Work out the finished part from the listing and answer in its coordinate system (mm). A direction names the side the tool comes from. Round coordinates to 2 decimals unless told otherwise and drop trailing zeros. Write each loop counter-clockwise with the first axis right and the second up, starting at its lowest first coordinate (ties: lowest second). Pieces come first, ordered by that corner, then holes. Notation, with made-up numbers: (39.5, 7) -> (47.5, 7) arc R28 cw to (47.5, 41) -> close; hole circle Ø5 at (55.25, 46.5). An arc over 180 degrees is marked (long way). Answer as a JSON object with one key per item and string values. Group by question number.
from build123d import *

# Parameters (mm, degrees)
SKETCH_1_W               = 5.5
SKETCH_1_H               = 9.9
EXTRUDE_1_DEPTH          = 6.44
SKETCH_2_W               = 1.5
SKETCH_2_H               = 0.15
PATTERN_LINEAR_1_COUNT   = 2
PATTERN_LINEAR_1_PITCH   = 2.54
SKETCH_3_W               = 1.5
SKETCH_3_H               = 0.15
PATTERN_LINEAR_2_COUNT   = 2
PATTERN_LINEAR_2_PITCH   = 2.54
CUT_EXTRUDE_1_DEPTH      = 0.15
CUT_EXTRUDE_1_DEPTH_BACK = 0.15
CUT_EXTRUDE_4_DEPTH      = 0.15
CUT_EXTRUDE_4_DEPTH_BACK = 0.15
CUT_EXTRUDE_5_DEPTH      = 0.15
CUT_EXTRUDE_5_DEPTH_BACK = 0.15
CUT_EXTRUDE_6_DEPTH      = 0.15
CUT_EXTRUDE_6_DEPTH_BACK = 0.15
SKETCH_6_W               = 1.4
SKETCH_6_H               = 3.5
CUT_EXTRUDE_1_2_DEPTH    = 1
PATTERN_LINEAR_3_COUNT   = 2
PATTERN_LINEAR_3_PITCH   = 2.54
EXTRUDE_2_DEPTH          = 2
SKETCH_8_W               = 5.49587381
SKETCH_8_H               = 0.4
EXTRUDE_3_DEPTH          = 0.4
FILLET_1_R               = 0.08


with BuildPart() as part:
    # Эскиз1 → Вытянуть1 (new body)
    with BuildSketch(Plane(origin=(0, 0, 0), x_dir=(0, 0, -1), z_dir=(1, 0, 0))):
        Rectangle(SKETCH_1_W, SKETCH_1_H)
    extrude(amount=EXTRUDE_1_DEPTH)

    # По траектории1: sweep along a curve in space
    with BuildLine() as sweep_1_path:
        Line((4.49, 3.95, -2.75), (4.49, 3.95, -3.790830974))
        ThreePointArc((4.49, 3.95, -3.790830974), (4.49, 3.906490428, -3.915373119), (4.49, 3.794892541, -3.98572751))
        Line((4.49, 3.794892541, -3.98572751), (4.49, -3.95, -5.769688961))
        Line((4.49, -3.95, -5.769688961), (4.49, -7.85, -5.769688961))
    # Эскиз2 → По траектории1 (sweep)
    with BuildSketch(Plane(origin=(0, 0, -2.75), x_dir=(-1, 0, 0), z_dir=(0, 0, -1))):
        with Locations((-4.49, 3.95)):
            Rectangle(SKETCH_2_W, SKETCH_2_H)
    sweep_1 = sweep(path=sweep_1_path.line, transition=Transition.RIGHT)

    # Линейный массив1: По траектории1 ×2
    with Locations(*[(-i * PATTERN_LINEAR_1_PITCH, 0, 0) for i in range(1, PATTERN_LINEAR_1_COUNT)]):
        add(sweep_1)

    # По траектории2: sweep along a curve in space
    with BuildLine() as sweep_2_path:
        Line((4.49, -3.95, -2.75), (4.49, -3.95, -4.02144183))
        ThreePointArc((4.49, -3.95, -4.02144183), (4.49, -4.008578644, -4.162863187), (4.49, -4.15, -4.22144183))
        Line((4.49, -4.15, -4.22144183), (4.49, -7.85, -4.22144183))
    # Эскиз3 → По траектории2 (sweep)
    with BuildSketch(Plane(origin=(0, 0, -2.75), x_dir=(-1, 0, 0), z_dir=(0, 0, -1))):
        with Locations((-4.49, -3.95)):
            Rectangle(SKETCH_3_W, SKETCH_3_H)
    sweep_2 = sweep(path=sweep_2_path.line)

    # Линейный массив2: По траектории2 ×2
    with Locations(*[(-i * PATTERN_LINEAR_2_PITCH, 0, 0) for i in range(1, PATTERN_LINEAR_2_COUNT)]):
        add(sweep_2)

    # Эскиз4 → Cut-Extrude 1 (cut, two sides: drawn at the far end of the back side and taken through both)
    with BuildSketch(Plane(origin=(0, 0, -5.844688961), x_dir=(-1, 0, 0), z_dir=(0, 0, -1)).offset(-CUT_EXTRUDE_1_DEPTH_BACK)):
        Polygon((-1.21347651, -4.143413371), (-1.665, -5.067248723), (-1.665, -6.848447142), (-1.871476359, -7.835), (-2.028523641, -7.835), (-2.235, -6.848447142), (-2.235, -5.067248723), (-2.68652349, -4.143413371), (-2.71347651, -4.156586629), (-2.265, -5.074187736), (-2.265, -6.851552858), (-2.052894917, -7.865), (-1.847105083, -7.865), (-1.635, -6.851552858), (-1.635, -5.074187736), (-1.18652349, -4.156586629), align=None)
    extrude(amount=CUT_EXTRUDE_1_DEPTH + CUT_EXTRUDE_1_DEPTH_BACK, mode=Mode.SUBTRACT)


with BuildPart() as cut_extrude_1_kept_piece:
    # of the separate pieces the step leaves, the one the design keeps (cut_extrude_1_pieces_kept)
    add(part.part.solids().sort_by_distance((0, 4.95, 2.75))[0])

    # Эскиз4<4> → Вырез-Вытянуть-Тонкостенный4 (cut, two sides: drawn at the far end of the back side and taken through both)
    with BuildSketch(Plane(origin=(0, 0, -5.844688961), x_dir=(-1, 0, 0), z_dir=(0, 0, -1)).offset(-CUT_EXTRUDE_4_DEPTH_BACK)):
        Polygon((-1.21347651, -4.143413371), (-1.665, -5.067248723), (-1.665, -6.848447142), (-1.871476359, -7.835), (-2.028523641, -7.835), (-2.235, -6.848447142), (-2.235, -5.067248723), (-2.68652349, -4.143413371), (-2.71347651, -4.156586629), (-2.265, -5.074187736), (-2.265, -6.851552858), (-2.052894917, -7.865), (-1.847105083, -7.865), (-1.635, -6.851552858), (-1.635, -5.074187736), (-1.18652349, -4.156586629), align=None)
        Polygon((-5.25347651, -4.156586629), (-4.805, -5.074187736), (-4.805, -6.851558008), (-4.592177182, -7.865), (-4.387822818, -7.865), (-4.175, -6.851558008), (-4.175, -5.074187736), (-3.72652349, -4.156586629), (-3.75347651, -4.143413371), (-4.205, -5.067248723), (-4.205, -6.848441992), (-4.412177182, -7.835), (-4.567822818, -7.835), (-4.775, -6.848441992), (-4.775, -5.067248723), (-5.22652349, -4.143413371), align=None)
    extrude(amount=CUT_EXTRUDE_4_DEPTH + CUT_EXTRUDE_4_DEPTH_BACK, mode=Mode.SUBTRACT)


with BuildPart() as cut_extrude_4_kept_piece:
    # of the separate pieces the step leaves, the one the design keeps (cut_extrude_4_pieces_kept)
    add(cut_extrude_1_kept_piece.part.solids().sort_by_distance((0, 4.95, 2.75))[0])

    # Эскиз5 → Вырез-Вытянуть-Тонкостенный5 (cut, two sides: drawn at the far end of the back side and taken through both)
    with BuildSketch(Plane.XY.offset(-4.14644183).offset(-CUT_EXTRUDE_5_DEPTH_BACK)):
        Polygon((1.18652349, -4.156586629), (1.635, -5.074187736), (1.635, -6.851552858), (1.847105083, -7.865), (2.052894917, -7.865), (2.265, -6.851552858), (2.265, -5.074187736), (2.71347651, -4.156586629), (2.68652349, -4.143413371), (2.235, -5.067248723), (2.235, -6.848447142), (2.028523641, -7.835), (1.871476359, -7.835), (1.665, -6.848447142), (1.665, -5.067248723), (1.21347651, -4.143413371), align=None)
    extrude(amount=CUT_EXTRUDE_5_DEPTH + CUT_EXTRUDE_5_DEPTH_BACK, mode=Mode.SUBTRACT)


with BuildPart() as cut_extrude_5_kept_piece:
    # of the separate pieces the step leaves, the one the design keeps (cut_extrude_5_pieces_kept)
    add(cut_extrude_4_kept_piece.part.solids().sort_by_distance((0, 4.95, 2.75))[0])

    # Эскиз5<4> → Вырез-Вытянуть-Тонкостенный6 (cut, two sides: drawn at the far end of the back side and taken through both)
    with BuildSketch(Plane.XY.offset(-4.14644183).offset(-CUT_EXTRUDE_6_DEPTH_BACK)):
        Polygon((1.18652349, -4.156586629), (1.635, -5.074187736), (1.635, -6.851552858), (1.847105083, -7.865), (2.052894917, -7.865), (2.265, -6.851552858), (2.265, -5.074187736), (2.71347651, -4.156586629), (2.68652349, -4.143413371), (2.235, -5.067248723), (2.235, -6.848447142), (2.028523641, -7.835), (1.871476359, -7.835), (1.665, -6.848447142), (1.665, -5.067248723), (1.21347651, -4.143413371), align=None)
        Polygon((5.22652349, -4.143413371), (4.775, -5.067248723), (4.775, -6.848441992), (4.567822818, -7.835), (4.412177182, -7.835), (4.205, -6.848441992), (4.205, -5.067248723), (3.75347651, -4.143413371), (3.72652349, -4.156586629), (4.175, -5.074187736), (4.175, -6.851558008), (4.387822818, -7.865), (4.592177182, -7.865), (4.805, -6.851558008), (4.805, -5.074187736), (5.25347651, -4.156586629), align=None)
    extrude(amount=CUT_EXTRUDE_6_DEPTH + CUT_EXTRUDE_6_DEPTH_BACK, mode=Mode.SUBTRACT)


with BuildPart() as cut_extrude_6_kept_piece:
    # of the separate pieces the step leaves, the one the design keeps (cut_extrude_6_pieces_kept)
    add(cut_extrude_5_kept_piece.part.solids().sort_by_distance((0, 4.95, 2.75))[0])

    # Эскиз6 → Cut-Extrude 1 2 (cut)
    with BuildSketch(Plane.XY.offset(2.75)):
        with Locations((2.004611319, 0)):
            Rectangle(SKETCH_6_W, SKETCH_6_H)
    cut_extrude_1_2 = extrude(amount=-CUT_EXTRUDE_1_2_DEPTH, mode=Mode.SUBTRACT)

    # Линейный массив3: Cut-Extrude 1 2 ×2
    with Locations(*[(i * PATTERN_LINEAR_3_PITCH, 0, 0) for i in range(1, PATTERN_LINEAR_3_COUNT)]):
        add(cut_extrude_1_2, mode=Mode.SUBTRACT)

    # Эскиз7 → Вытянуть2 (add)
    with BuildSketch(Plane.XY.offset(1.75)):
        with BuildLine():
            Line((1.304611319, -0.15), (1.304611319, -1.75))
            ThreePointArc((1.304611319, -1.75), (2.004611319, -1.460050506), (2.704611319, -1.75))
            Line((2.704611319, -1.75), (2.704611319, -0.15))
            ThreePointArc((2.704611319, -0.15), (2.004611319, -0.439949494), (1.304611319, -0.15))
        make_face()
        with BuildLine():
            Line((3.844611319, -0.15), (3.844611319, -1.75))
            ThreePointArc((3.844611319, -1.75), (4.544611319, -1.460050506), (5.244611319, -1.75))
            Line((5.244611319, -1.75), (5.244611319, -0.15))
            ThreePointArc((5.244611319, -0.15), (4.544611319, -0.439949494), (3.844611319, -0.15))
        make_face()
    extrude(amount=EXTRUDE_2_DEPTH)

    # Эскиз8 → Вытянуть3 (add)
    with BuildSketch(Plane(origin=(0, 0, -2.75), x_dir=(-1, 0, 0), z_dir=(0, 0, -1))):
        with Locations((-3.22, 2.2)):
            Rectangle(SKETCH_8_W, SKETCH_8_H)
        with Locations((-3.22, -2.2)):
            Rectangle(SKETCH_8_W, SKETCH_8_H)
    extrude(amount=EXTRUDE_3_DEPTH)

    # Скругление1
    fillet_1_edges = [cut_extrude_6_kept_piece.edges().sort_by_distance(p)[0] for p in [
        (0, 0, -2.75),
        (3.22, -4.95, -2.75),
        (0, 0, 2.75),
        (3.22, 4.95, 2.75),
        (0, -4.95, 0),
        (3.22, -4.95, 2.75),
        (0, 4.95, 0),
        (3.22, 4.95, -2.75),
        (6.44, 0, 2.75),
        (6.44, -4.95, 0),
        (6.44, 0, -2.75),
        (6.44, 4.95, 0),
    ]]
    fillet(fillet_1_edges, radius=FILLET_1_R)


solid = cut_extrude_6_kept_piece.part
1) A cutting plane is placed at D-D on z = 2. Determine the outline of the cut face in (x, y).
2) A cutting plane is placed at B-B on y = -5.5. Determine the outline of the cut face in (x, z) (3 decimals).
3) For a pull along Y with two mould halves and no side action, classify faces 5 (the face through (3, 0, 2.75)), 6 (the face through (4, 4.025, -3)), 7 (the face through (4.53, -1.46, 2.74)) as released by +Y, released by -Y, zero draft, split by the parting line, or undercut.
4) A cutting plane is placed at C-C on y = -3.5. Determine the outline of the cut face in (x, z).
5) Each of these flat-tipped pins is pushed along its axis until it touches: P1, Ø1.5, axis at y = 1, z = -5, coming from the +X side; P2, Ø1, axis at x = 4, z = -3.5, coming from the -Y side (3 decimals); P3, Ø1.5, axis at x = 2, y = 1, coming from the +Z side. Where does it stop, or does it pass through?
6) A tool of negligible diameter and unlimited length cuts with its end or side. For faces 1 (the face through (5.245, -1, 3)), 2 (the face through (5, 3.875, -3)), 3 (the face through (2, 4.025, -3)), 4 (the face through (2, 1.75, 2)), from which of +Z, -Z, +X, -X, +Y, -Y can it reach the whole face along a straight path? Write none if from no direction.
7) A cutting plane is placed at A-A on z = -3.5. Determine the outline of the cut face in (x, y) (3 decimals).
8) Straight lines are drawn through the part: L1, parallel to Z at x = 5, y = -4.5; L2, parallel to Y at x = 5.25, z = -0.5; L3, parallel to Z at x = 5.5, y = 3.5. For each, find the intervals that lie inside material, in ascending order.
Established:
{
 "1": {"outline": "(0, -4.87) arc R0.08 ccw to (0.08, -4.95) -> (6.36, -4.95) arc R0.08 ccw to (6.44, -4.87) -> (6.44, 4.87) arc R0.08 ccw to (6.36, 4.95) -> (0.08, 4.95) arc R0.08 ccw to (0, 4.87) -> close; hole (1.3, -1.75) -> (2.7, -1.75) arc R0.99 ccw to start; hole (1.3, -0.15) arc R0.99 ccw to (2.7, -0.15) -> (2.7, 1.75) -> (1.3, 1.75) -> close; hole (3.84, -1.75) -> (5.24, -1.75) arc R0.99 ccw to start; hole (3.84, -0.15) arc R0.99 ccw to (5.24, -0.15) -> (5.24, 1.75) -> (3.84, 1.75) -> close"},
 "2": {"outline": "(1.665, -5.845) -> (2.235, -5.845) -> (2.235, -5.695) -> (1.665, -5.695) -> close; (1.665, -4.296) -> (2.235, -4.296) -> (2.235, -4.146) -> (1.665, -4.146) -> close; (4.205, -5.845) -> (4.775, -5.845) -> (4.775, -5.695) -> (4.205, -5.695) -> close; (4.205, -4.296) -> (4.775, -4.296) -> (4.775, -4.146) -> (4.205, -4.146) -> close"},
 "3": {"face 5": "zero draft", "face 6": "released by +Y", "face 7": "undercut"},
 "4": {"outline": "(0, -2.67) arc R0.08 ccw to (0.08, -2.75) -> (6.36, -2.75) arc R0.08 ccw to (6.44, -2.67) -> (6.44, 2.67) arc R0.08 ccw to (6.36, 2.75) -> (0.08, 2.75) arc R0.08 ccw to (0, 2.67) -> close; (1.2, -5.74) -> (2.7, -5.74) -> (2.7, -5.59) -> (1.2, -5.59) -> close; (3.74, -5.74) -> (5.24, -5.74) -> (5.24, -5.59) -> (3.74, -5.59) -> close"},
 "5": {"P1": "stops at x = 5.24", "P2": "stops at y = -4.025", "P3": "stops at z = 2.75"},
 "6": {"face 1": "+Z, +X, +Y, -Y", "face 2": "+X, -X", "face 3": "-Z, +X, -X, +Y", "face 4": "+Z"},
 "7": {"outline": "(1.2, -4.025) -> (2.7, -4.025) -> (2.7, -3.875) -> (1.2, -3.875) -> close; (1.2, 3.875) -> (2.7, 3.875) -> (2.7, 4.025) -> (1.2, 4.025) -> close; (3.74, -4.025) -> (5.24, -4.025) -> (5.24, -3.875) -> (3.74, -3.875) -> close; (3.74, 3.875) -> (5.24, 3.875) -> (5.24, 4.025) -> (3.74, 4.025) -> close"},
 "8": {"L1": "z = -5.84 to -5.69, -4.3 to -4.15, -2.75 to 2.75", "L2": "y = -4.95 to 4.95", "L3": "z = -2.75 to 2.75"}
}
